For this review, take the finished solid that the model builds, in its own axes (mm). Face numbers are marked on the shaded views. A direction names the side the tool comes from. Coordinates: 2 decimals unless noted, no trailing zeros. Loops run counter-clockwise (first coordinate to the right, second up) from the corner with the lowest first, then second, coordinate; pieces in that order, holes last. Notation, with made-up numbers: (7.25, -16) -> (34.25, -16) arc R8 ccw to (34.25, -4) -> close; hole circle Ø2 at (35.25, -8). An arc over 180 degrees is marked (long way). Use a Markdown table: item, result.
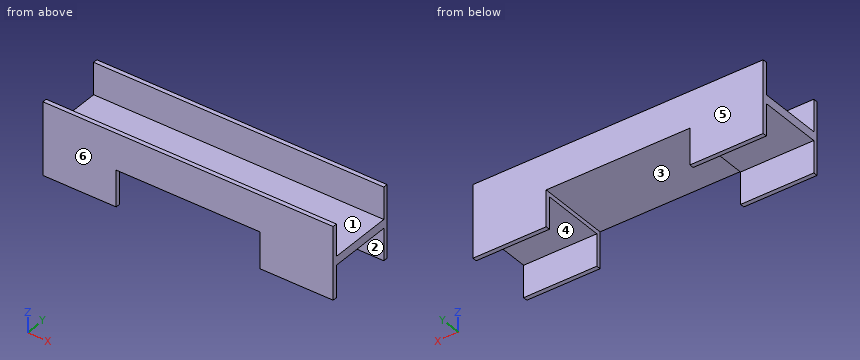
from build123d import *

# Parameters (mm, degrees)
F0_W     = 200
F0_H     = 25
F1_DEPTH = 50
F2_W     = 44
F2_H     = 22
F3_DEPTH = 100.001
F4_DEPTH = 100.001
F5_W     = 50.4667520523
F5_H     = 50
F6_DEPTH = 25
F8_DEPTH = 200.001


with BuildPart() as f1:
    # F0 (on Front) → F1 (new body)
    with BuildSketch(Plane.XZ):
        Rectangle(F0_W, F0_H)
    extrude(amount=F1_DEPTH)

    # F2 (on Right) → F3 (cut, through all)
    with BuildSketch(Plane.YZ):
        with Locations((-25, 1.5)):
            Rectangle(F2_W, F2_H)
    extrude(amount=F3_DEPTH, mode=Mode.SUBTRACT)

    # F2 (on Right) → F4 (cut, through all)
    with BuildSketch(Plane.YZ):
        with Locations((-25, 1.5)):
            Rectangle(F2_W, F2_H)
    extrude(amount=-F4_DEPTH, mode=Mode.SUBTRACT)

    # F5 (on face) → F6 (join)
    with BuildSketch(Plane(origin=(0, 0, -12.5), x_dir=(1, 0, 0), z_dir=(0, 0, -1))):
        with Locations((74.7666239738, 25)):
            Rectangle(F5_W, F5_H)
    extrude(amount=F6_DEPTH)

    # F7 (on face) → F8 (cut, through all)
    with BuildSketch(Plane.YZ.offset(100)):
        Polygon((-47, -31.9465436041), (-47, -37.5), (-3, -37.5), (-3, -31.9465436041), (-3, -15.5), (-24.8005185276, -15.5), (-47, -15.5), align=None)
    extrude(amount=-F8_DEPTH, mode=Mode.SUBTRACT)

    # F9: F1 across plane


with BuildPart() as f1_1:
    add(f1.part)
    add(f1.part.mirror(Plane.YZ))


solid = f1_1.part
(1) Mouldability with a two-part tool opening along Y and no side actions: class the marked faces 4, 5 and 6 as pulls with the +Y half, pulls with the -Y half, needs draft (parallel to the pull), parting line crosses it, or undercut.
Found:
| item | result |
|---|---|
| face 4 | undercut |
| face 5 | pulls with the +Y half |
| face 6 | pulls with the -Y half |
(2) Take a section at B-B on x = -16. Write out the cut boundary in (y, z).
Found:
| item | result |
|---|---|
| outline | (-50, -12.5) -> (0, -12.5) -> (0, 12.5) -> (-3, 12.5) -> (-3, -9.5) -> (-47, -9.5) -> (-47, 12.5) -> (-50, 12.5) -> close |
(3) Take a section at D-D on z = 4. Write out the cut boundary in (x, y), plus the area to 3 significant figures.
Found:
| item | result |
|---|---|
| outline | (-100, -50) -> (100, -50) -> (100, -47) -> (-100, -47) -> close; (-100, -3) -> (100, -3) -> (100, 0) -> (-100, 0) -> close |
| area | 1,200 mm^2 |
(4) For the marked faces 1, 2 and 3, list the 3-axis set-ups (+Z, -Z, +X, -X, +Y, -Y) from which the entire face can be reached by the end or side of a thin tool; tool diameter is ignored.
Found:
| item | result |
|---|---|
| face 1 | +Z, +X, -X |
| face 2 | -Z, +X, -X |
| face 3 | -Z, +Y, -Y |
(5) Take a section at C-C on y = -40. Write out the cut boundary in (x, z).
Found:
| item | result |
|---|---|
| outline | (-100, -15.5) -> (-49.53, -15.5) -> (-49.53, -12.5) -> (49.53, -12.5) -> (49.53, -15.5) -> (100, -15.5) -> (100, -9.5) -> (-100, -9.5) -> close |
(6) For line 1 along Y through (x, z) = (57, -24.5); line 2 along X through (y, z) = (-40.5, -14); line 3 along Z through (x, y) = (-32, -18), list the stretches that pass through material, from the lowest coordinate up.
Found:
| item | result |
|---|---|
| line 1 | y = -50 to -47, -3 to 0 |
| line 2 | x = -100 to -49.53, 49.53 to 100 |
| line 3 | z = -12.5 to -9.5 |
(7) For pin 1 Ø22 at (x, y) = (66, -27.5) entering from -Z; pin 2 Ø4 at (x, y) = (-35.5, -38.5) entering from +Z; pin 3 Ø15 at (x, y) = (7, -27.5) entering from -Z, all flat-tipped, find the tip position at first contact; note any pin that passes through.
Found:
| item | result |
|---|---|
| pin 1 | stops at z = -15.5 |
| pin 2 | stops at z = -9.5 |
| pin 3 | stops at z = -12.5 |
(8) Take a section at A-A on z = -26. Write out the cut boundary in (x, y), plus the area to 3 significant figures.
Found:
| item | result |
|---|---|
| outline | (-100, -50) -> (-49.53, -50) -> (-49.53, -47) -> (-100, -47) -> close; (-100, -3) -> (-49.53, -3) -> (-49.53, 0) -> (-100, 0) -> close; (49.53, -50) -> (100, -50) -> (100, -47) -> (49.53, -47) -> close; (49.53, -3) -> (100, -3) -> (100, 0) -> (49.53, 0) -> close |
| area | 606 mm^2 |
